Work out the finished part from the listing and answer in its coordinate system (mm). A direction names the side the tool comes from. Coordinates: 2 decimals unless noted, no trailing zeros. Order: outer loops, then holes, each group sorted by start corner. A loop starts at its lowest first (then second) coordinate and runs counter-clockwise, first axis right, second up. Notation, with made-up numbers: M 87.25,52 L 122.25,52 A12 ccw 122.25,73 Z; hole C 82.5,-4 d9. An arc over 180 degrees is marked long. Use a Markdown table: item, result.
from build123d import *

# Parameters (mm, degrees)
BOSS_EXTRU_1_DEPTH      = 110
ESQUISSE2_R             = 1.5
ENL_V_MAT_EXTRU_1_DEPTH = 5
CHANFREIN1_SIZE         = 1


with BuildPart() as part:
    # Esquisse1 → Boss.-Extru.1 (new body)
    with BuildSketch(Plane.XY):
        with BuildLine():
            Line((0, 0.5), (0, 9.25))
            Line((0, 9.25), (1, 9.25))
            Line((1, 9.25), (1, 1.5))
            ThreePointArc((1, 1.5), (1.146446609, 1.146446609), (1.5, 1))
            Line((1.5, 1), (11.5, 1))
            Line((11.5, 1), (11.5, 0))
            Line((11.5, 0), (0.5, 0))
            ThreePointArc((0.5, 0), (0.146446609, 0.146446609), (0, 0.5))
        make_face()
    extrude(amount=BOSS_EXTRU_1_DEPTH)

    # Esquisse2 → Enlèv. mat.-Extru.1 (cut)
    with BuildSketch(Plane.XZ):
        with Locations((5.2, 5)):
            Circle(ESQUISSE2_R)
        with Locations((5.2, 105)):
            Circle(ESQUISSE2_R)
    extrude(amount=-ENL_V_MAT_EXTRU_1_DEPTH, mode=Mode.SUBTRACT)

    # Chanfrein1
    chanfrein1_edges = [part.edges().sort_by_distance(p)[0] for p in [
        (3.7, 0, 5),
        (3.7, 0, 105),
    ]]
    chamfer(chanfrein1_edges, length=CHANFREIN1_SIZE - 0.0001)  # a hair under: the kernel refuses the full size


solid = part.part
1. Section D-D on y = 5.5 is taken. Determine the outline of the cut face in (x, z), then the cut area to 3 significant figures.
Answers below:
| item | result |
|---|---|
| outline | M 0,0 L 1,0 L 1,110 L 0,110 Z |
| area | 110 mm² |
2. Find the intervals of material crossed by probe 1 along Y at (x, z) = (10.25, 103.5), in increasing order.
Answers below:
| item | result |
|---|---|
| probe 1 | 0 to 1 |
3. Section C-C on z = 62 is taken. Determine the outline of the cut face in (x, y).
Answers below:
| item | result |
|---|---|
| outline | M 0,0.5 A0.5 ccw 0.5,0 L 11.5,0 L 11.5,1 L 1.5,1 A0.5 cw 1,1.5 L 1,9.25 L 0,9.25 Z |
4. Section A-A on x = 5.2 is taken. Give the number of separate pieces and of enclosed holes in the cut face, then the cut area to 3 significant figures.
Answers below:
| item | result |
|---|---|
| separate pieces | 3 |
| enclosed holes | 0 |
| area | 102 mm² |
5. Flat-ended cylindrical pins translate along their axes: P1, Ø4, axis at x = 5.2, z = 5, coming from the -Y side; P2, Ø1, axis at x = 9.5, z = 69.5, coming from the +Y side; P3, Ø2, axis at y = 4.5, z = 83, coming from the +X side; P4, Ø5, axis at y = 3, z = 94, coming from the -X side. Find the tip coordinate at first contact, or state that the pin passes through.
Answers below:
| item | result |
|---|---|
| P1 | y = 0.5 |
| P2 | y = 1 |
| P3 | x = 1 |
| P4 | x = 0 |
6. For faces 1 (the face through (6, 1, 54)), 2 (the face through (3.2, 0.5, 0)), determine the directions among +Z, -Z, +X, -X, +Y, -Y from which every point of the face is accessible in a straight line to the end or side of a thin tool.
Answers below:
| item | result |
|---|---|
| face 1 | +Z, -Z, +X, +Y |
| face 2 | -Z, +X, -X, +Y, -Y |
